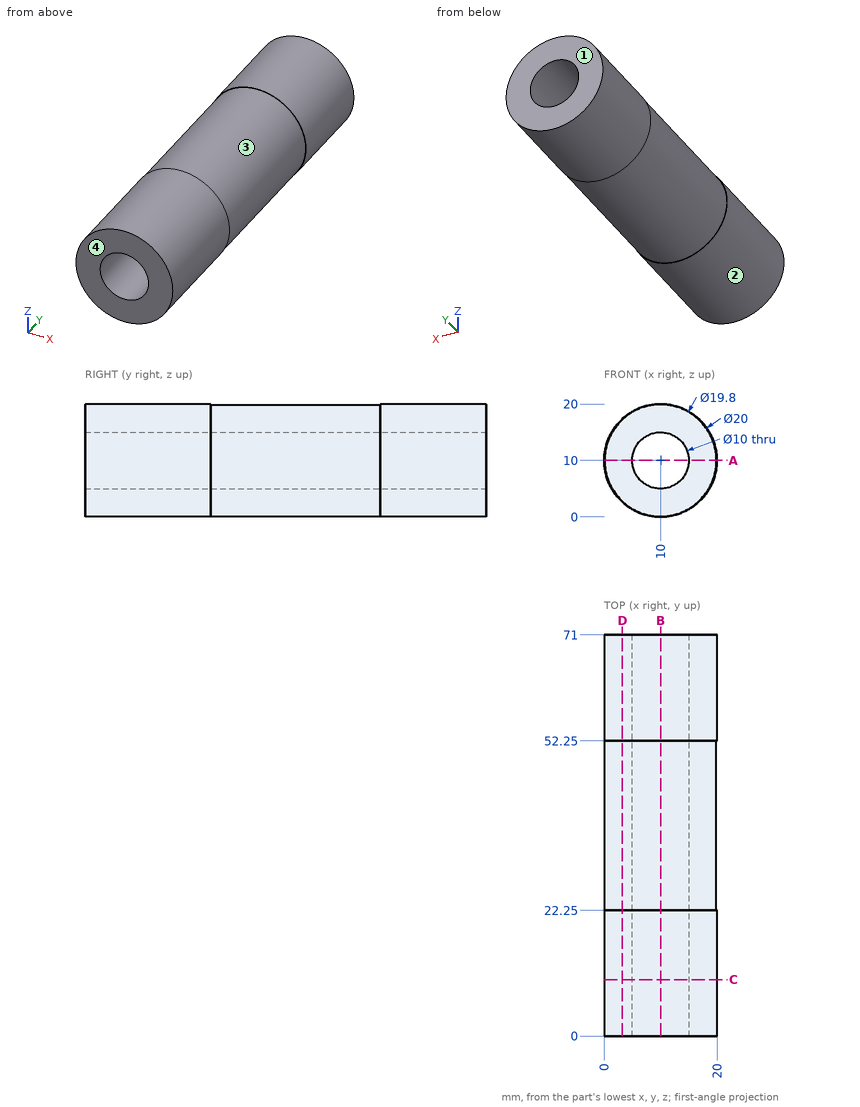
Verification items for this drawing (mm, ordinates from the low corner). Give positions to 0.01 mm unless a question says otherwise; leave off trailing zeros. Order: outer loops, then holes, each group sorted by start corner. A loop starts at its lowest first (then second) coordinate and runs counter-clockwise, first axis right, second up. Notation, with made-up numbers: M 50,71.5 L 97,71.5 A10 ccw 97,87.5 Z; hole C 80.25,-7.5 d8. An arc over 180 degrees is marked long. Use a Markdown table: item, result.
Item 1: Section check C-C (y = 10). Record the cut outline in (x, z), and give its area (3 significant figures).
Answers follow:
| item | result |
|---|---|
| outline | C 10,10 d20; hole C 10,10 d10 |
| area | 236 mm2 |
Item 2: Draft check along Y on the marked faces 1, 2, 3 and 4. Enter one of: +Y half, -Y half, draft (parallel to the pull), parting line (faces both ways), or undercut.
Answers follow:
| item | result |
|---|---|
| face 1 | +Y half |
| face 2 | draft |
| face 3 | undercut |
| face 4 | -Y half |
Item 3: Section check A-A (z = 10). Record the cut outline in (x, y).
Answers follow:
| item | result |
|---|---|
| outline | M 0,0 L 5,0 L 5,71 L 0,71 L 0,52.25 L 0.1,52.25 L 0.1,22.25 L 0,22.25 Z; M 15,0 L 20,0 L 20,22.25 L 19.9,22.25 L 19.9,52.25 L 20,52.25 L 20,71 L 15,71 Z |
Item 4: Depth check by flat-ended pin: P1, Ø2, axis at x = 7.5, y = 25, coming from the +Z side; P2, Ø6, axis at y = 32.5, z = 16, coming from the +X side; P3, Ø1, axis at y = 33, z = 15.5, coming from the -X side. Enter the tip coordinate at first touch or a pass-through.
Answers follow:
| item | result |
|---|---|
| P1 | stops at z = 19.79 |
| P2 | stops at x = 19.43 |
| P3 | stops at x = 1.46 |
Item 5: Material ranges on line 1 along X through (y, z) = (54.5, 10); line 2 along X through (y, z) = (49.5, 13), recorded low to high.
Answers follow:
| item | result |
|---|---|
| line 1 | x = 0 to 5, 15 to 20 |
| line 2 | x = 0.57 to 6, 14 to 19.43 |
Item 6: Section check D-D (x = 3.25). Record the cut outline in (y, z).
Answers follow:
| item | result |
|---|---|
| outline | M 0,2.62 L 22.25,2.62 L 22.25,2.76 L 52.25,2.76 L 52.25,2.62 L 71,2.62 L 71,17.38 L 52.25,17.38 L 52.25,17.24 L 22.25,17.24 L 22.25,17.38 L 0,17.38 Z |
Item 7: Section check B-B (x = 10). Record the cut outline in (y, z).
Answers follow:
| item | result |
|---|---|
| outline | M 0,0 L 22.25,0 L 22.25,0.1 L 52.25,0.1 L 52.25,0 L 71,0 L 71,5 L 0,5 Z; M 0,15 L 71,15 L 71,20 L 52.25,20 L 52.25,19.9 L 22.25,19.9 L 22.25,20 L 0,20 Z |
